The listing builds one solid part. Answer for the finished solid, in the listing's coordinates (mm). A direction names the side the tool comes from. Give positions to 0.01 mm unless a question says otherwise; leave off trailing zeros. Order: outer loops, then holes, each group sorted by start corner. A loop starts at its lowest first (then second) coordinate and runs counter-clockwise, first axis right, second up. Notation, with made-up numbers: (41.5, 5.25) - (63.5, 5.25) arc R32 cw to (63.5, 34.25) - close; hole circle Ø3 at (24, 12.25). An arc over 180 degrees is marked (long way). Answer as CSV lines item,"result". Start each with the question number.
1. Section A-A on y = 13.5 is taken. Give the vertices of the cut face in (x, z).
2. Consider line 1 along X through (y, z) = (15.75, 2.75); line 2 along X through (y, z) = (15.75, 1.9); line 3 along Z through (x, y) = (-25, 12.5). Determine where each line is inside the solid, lowest interval first. Write a range as [from, to].
3. Section D-D on x = -28 is taken. Give the vertices of the cut face in (y, z).
4. Which of the six approach directions +Z, -Z, +X, -X, +Y, -Y give full straight-line access (tool end or side, diameter ignored) to faces 5 (the cylindrical face through (-24.1, 18.34, 2.76)), 6 (the cylindrical face through (-33.85, 15.63, 1.18))?
5. Determine the mould class of faces 1 (the cylindrical face through (-21.611, 13.563, 1.553)), 2 (the flat face through (-26, 10.878, 1)), 3 (the flat face through (-26, 20.53, 1)), 4 (the flat face through (-26, 16, 0)) for opening direction Y: +Y half, -Y half, draft (parallel to the pull), parting line (faces both ways), or undercut.
6. A flat-ended cylindrical pin translates along its axis: pin 1 (4 mm diameter, centred on x = -31, y = 13.5, fed in from +Z). Find the tip coordinate at first contact, or state that the pin passes through.
7. Section B-B on x = -24.5 is taken. Give the vertices of the cut face in (y, z), and give its area (3 significant figures).
8. Section C-C on z = 1.6 is taken. Give the vertices of the cut face in (x, y), and give its area (3 significant figures).
from build123d import *

# Parameters (mm, degrees)
SKETCH1_R      = 2.413
EXTRUDE1_DEPTH = 2.3876
SKETCH2_R      = 2.9718
SKETCH2_R_2    = 2.413
EXTRUDE2_DEPTH = 0.762


with BuildPart() as part:
    # Sketch1 → Extrude1 (new body)
    with BuildSketch(Plane.XY):
        with BuildLine():
            Line((-32.197236546, 20.530230269), (-19.613461217, 20.530230269))
            ThreePointArc((-19.613461217, 20.530230269), (-17.9745326, 15.704230269), (-19.613461217, 10.878230269))
            Line((-19.613461217, 10.878230269), (-32.197236546, 10.878230269))
            ThreePointArc((-32.197236546, 10.878230269), (-33.8495326, 15.704230269), (-32.197236546, 20.530230269))
        make_face()
        with Locations((-22.7243326, 15.704230269)):
            Circle(SKETCH1_R, mode=Mode.SUBTRACT)
    extrude(amount=EXTRUDE1_DEPTH)

    # Sketch2 → Extrude2 (add)
    with BuildSketch(Plane.XY.offset(2.3876)):
        with Locations(Location((-22.7243326, 15.704230269, 0), (0, 0, 180))):
            Circle(SKETCH2_R)
        with Locations((-22.7243326, 15.704230269)):
            Circle(SKETCH2_R_2, mode=Mode.SUBTRACT)
    extrude(amount=EXTRUDE2_DEPTH)


solid = part.part
Checks:
1,outline,"(-33.53, 0) - (-23.71, 0) - (-23.71, 3.15) - (-24.72, 3.15) - (-24.72, 2.39) - (-33.53, 2.39) - close; (-21.74, 0) - (-18.29, 0) - (-18.29, 2.39) - (-20.73, 2.39) - (-20.73, 3.15) - (-21.74, 3.15) - close"
2,line 1,"x = [-25.7, -25.14], [-20.31, -19.75]"
2,line 2,"x = [-33.85, -25.14], [-20.31, -17.97]"
2,line 3,"z = [0, 2.39]"
3,outline,"(10.88, 0) - (20.53, 0) - (20.53, 2.39) - (10.88, 2.39) - close"
4,face 5,"+Z"
4,face 6,"+Z, -Z, -X"
5,face 1,"undercut"
5,face 2,"-Y half"
5,face 3,"+Y half"
5,face 4,"draft"
6,pin 1,"stops at z = 2.39"
7,outline,"(10.88, 0) - (14.07, 0) - (14.07, 3.15) - (13.32, 3.15) - (13.32, 2.39) - (10.88, 2.39) - close; (17.34, 0) - (20.53, 0) - (20.53, 2.39) - (18.09, 2.39) - (18.09, 3.15) - (17.34, 3.15) - close"
7,area,"16.4 mm²"
8,outline,"(-32.2, 10.88) - (-19.61, 10.88) arc R7.92 ccw to (-19.61, 20.53) - (-32.2, 20.53) arc R7.87 ccw to start; hole circle Ø4.83 at (-22.72, 15.7)"
8,area,"125 mm²"
